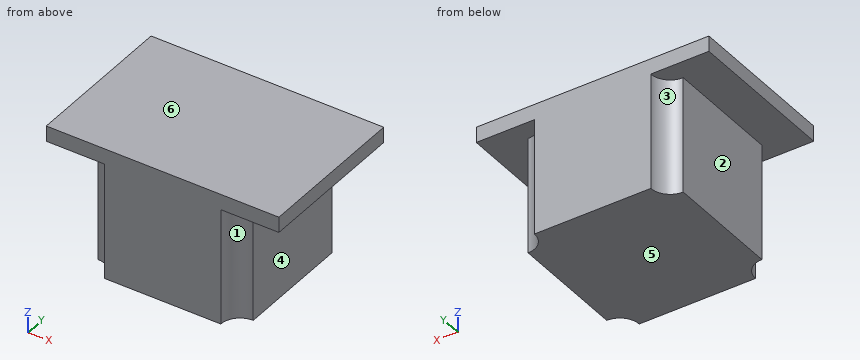
```python
from build123d import *

# Parameters (mm, degrees)
SKETCH1_W           = 300
SKETCH1_H           = 200
BOSS_EXTRUDE1_DEPTH = 20
SKETCH2_W           = 150
SKETCH2_H           = 25
SKETCH2_H_2         = 150
SKETCH2_W_2         = 25
BOSS_EXTRUDE2_DEPTH = 150
FILLET1_R           = 25
FILLET2_R           = 25


with BuildPart() as part:
    # Sketch1 → Boss-Extrude1 (new body)
    with BuildSketch(Plane.XY):
        Rectangle(SKETCH1_W, SKETCH1_H)
    extrude(amount=BOSS_EXTRUDE1_DEPTH)

    # Sketch2 → Boss-Extrude2 (add)
    with BuildSketch(Plane(origin=(0, 0, 0), x_dir=(-1, 0, 0), z_dir=(0, 0, -1))):
        with Locations((0, 87.5)):
            Rectangle(SKETCH2_W, SKETCH2_H)
        Rectangle(SKETCH2_W, SKETCH2_H_2)
        with Locations((-87.5, 0)):
            Rectangle(SKETCH2_W_2, SKETCH2_H_2)
        with Locations((87.5, 0)):
            Rectangle(SKETCH2_W_2, SKETCH2_H_2)
        with Locations((0, -87.5)):
            Rectangle(SKETCH2_W, SKETCH2_H)
    extrude(amount=BOSS_EXTRUDE2_DEPTH)

    # Fillet1
    fillet1_edges = [part.edges().sort_by_distance(p)[0] for p in [
        (75, 75, -75),
    ]]
    fillet(fillet1_edges, radius=FILLET1_R - 0.0001)  # a hair under: the kernel refuses the full size

    # Fillet2
    fillet2_edges = [part.edges().sort_by_distance(p)[0] for p in [
        (75, -75, -75),
        (-75, -75, -75),
        (-75, 75, -75),
    ]]
    fillet(fillet2_edges, radius=FILLET2_R - 0.0001)  # a hair under: the kernel refuses the full size


solid = part.part
```
Check sheet for the modelled part. Datum: model origin and axes. Units: mm. Face numbers are marked on the shaded views. A direction names the side the tool comes from. Give positions to 0.01 mm unless a question says otherwise; leave off trailing zeros. Write each loop counter-clockwise with the first axis right and the second up, starting at its lowest first coordinate (ties: lowest second). Pieces come first, ordered by that corner, then holes.
Item 1: Cross-section at C-C (x = 93.5). Enter the section's corners in (y, z), and give its area (3 significant figures).
Item 2: Scan lines: L1, parallel to X at y = -30, z = -45.5; L2, parallel to Z at x = -118.5, y = -26.5; L3, parallel to Y at x = 88.5, z = -27.5. Record each from-to range of solid material in increasing order.
Item 3: Cross-section at D-D (x = 125). Enter the section's corners in (y, z).
Item 4: Access from +Z, -Z, +X, -X, +Y, -Y to the whole of each face (thin tool, end or side, straight path). Record for the marked faces 1, 2 and 3.
Item 5: Draft check along Z on the marked faces 4, 5 and 6. Enter one of: released by +Z, released by -Z, zero draft, split by the parting line, or undercut.
Item 6: Gauge pin test, flat ends, axial feed: pin 1 (1.5 mm diameter, centred on y = 44.5, z = -59, fed in from +X); pin 2 (1 mm diameter, centred on y = -0.5, z = -108.5, fed in from -X). Record the tip position at first contact, or that the pin passes through.
Item 7: Cross-section at A-A (y = -3). Enter the section's corners in (x, z), and give its area (3 significant figures).
Report:
1. outline: (-100, 0) - (-75.86, 0) - (-75.86, -150) - (75.86, -150) - (75.86, 0) - (100, 0) - (100, 20) - (-100, 20) - close
1. area: 26,800 mm2
2. L1: x = -100 to 100
2. L2: z = 0 to 20
2. L3: y = -77.8 to 77.8
3. outline: (-100, 0) - (100, 0) - (100, 20) - (-100, 20) - close
4. face 1: -Z, +X, -Y
4. face 2: -Z, -X, +Y, -Y
4. face 3: -Z, -X, +Y
5. face 4: zero draft
5. face 5: released by -Z
5. face 6: released by +Z
6. pin 1: stops at x = 100
6. pin 2: stops at x = -100
7. outline: (-150, 0) - (-100, 0) - (-100, -150) - (100, -150) - (100, 0) - (150, 0) - (150, 20) - (-150, 20) - close
7. area: 36,000 mm2
